Source: three-view drawing plus pictorial views. Frame: mm from the lowest corner of the part. Give positions to 0.01 mm unless a question says otherwise; leave off trailing zeros. Write each loop counter-clockwise with the first axis right and the second up, starting at its lowest first coordinate (ties: lowest second). Pieces come first, ordered by that corner, then holes. Notation, with made-up numbers: (12, 18) -> (23, 18) arc R29 cw to (23, 55) -> close; hole circle Ø8 at (5, 42.25). An arc over 180 degrees is marked (long way). Write item = value, one per line.
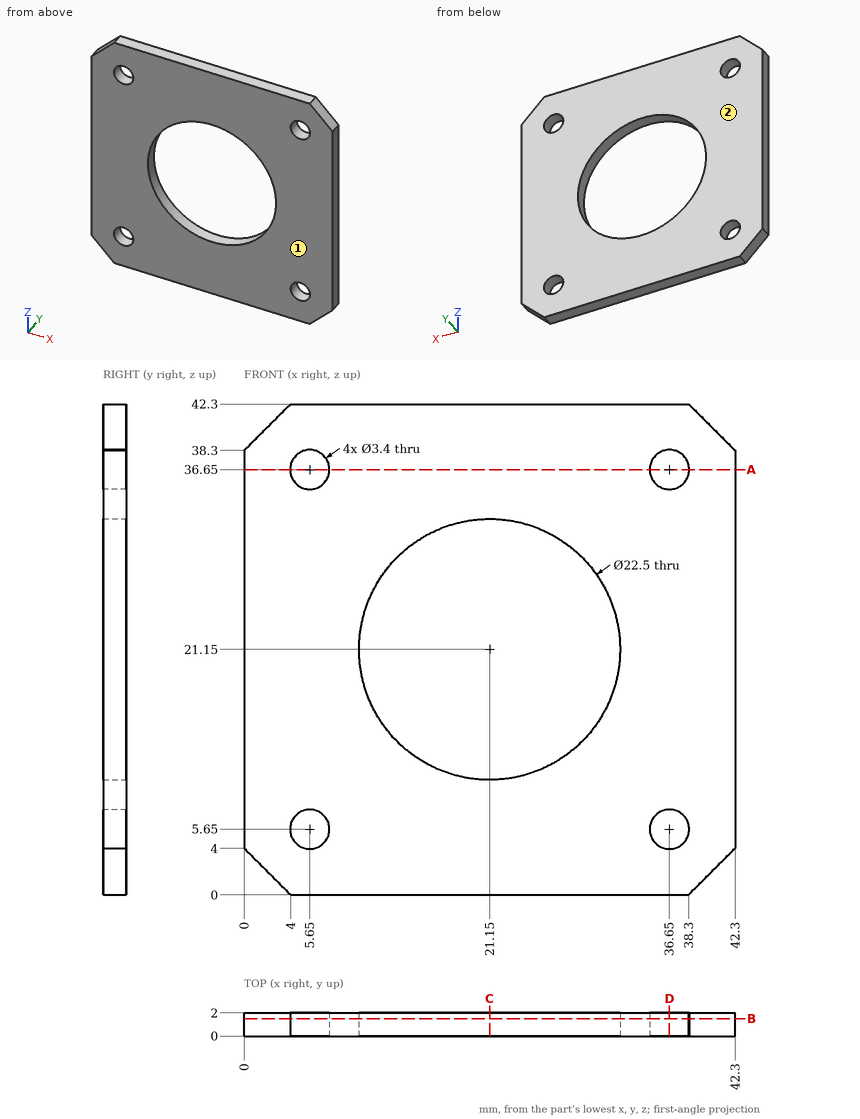
1) Cut plane D-D (x = 36.65). Return the cut outline in (y, z), then the cut area to 3 significant figures.
Computed:
outline = (0, 0) -> (2, 0) -> (2, 3.95) -> (0, 3.95) -> close; (0, 7.35) -> (2, 7.35) -> (2, 34.95) -> (0, 34.95) -> close; (0, 38.35) -> (2, 38.35) -> (2, 42.3) -> (0, 42.3) -> close
area = 71.0 mm²
2) Contact query for a flat-ended pin moving along its axis: pin 1 (2 mm diameter, centred on x = 5.65, z = 36.65, fed in from -Y). Output: stop coordinate, or through.
Computed:
pin_1 = through
3) Cut plane A-A (z = 36.65). Return the cut outline in (x, y), then the cut area to 3 significant figures.
Computed:
outline = (0, 0) -> (3.95, 0) -> (3.95, 2) -> (0, 2) -> close; (7.35, 0) -> (34.95, 0) -> (34.95, 2) -> (7.35, 2) -> close; (38.35, 0) -> (42.3, 0) -> (42.3, 2) -> (38.35, 2) -> close
area = 71.0 mm²
4) Material intervals for L1, parallel to Z at x = 5.65, y = 1.3; L2, parallel to X at y = 0.2, z = 21.5, sorted ascending.
Computed:
L1 = 0 to 3.95, 7.35 to 34.95, 38.35 to 42.3
L2 = 0 to 9.91, 32.39 to 42.3
5) Cut plane B-B (y = 1.5). Return the cut outline in (x, z), then the cut area to 3 significant figures.
Computed:
outline = (0, 4) -> (4, 0) -> (38.3, 0) -> (42.3, 4) -> (42.3, 38.3) -> (38.3, 42.3) -> (4, 42.3) -> (0, 38.3) -> close; hole circle Ø3.4 at (5.65, 5.65); hole circle Ø3.4 at (5.65, 36.65); hole circle Ø22.5 at (21.15, 21.15); hole circle Ø3.4 at (36.65, 5.65); hole circle Ø3.4 at (36.65, 36.65)
area = 1,320 mm²
6) Draft query along Y for the marked faces 1 and 2. Return one class per face: pulls with the +Y half, pulls with the -Y half, needs draft (parallel to the pull), parting line crosses it, or undercut.
Computed:
face_1 = pulls with the -Y half
face_2 = pulls with the +Y half
7) Cut plane C-C (x = 21.15). Return the cut outline in (y, z).
Computed:
outline = (0, 0) -> (2, 0) -> (2, 9.9) -> (0, 9.9) -> close; (0, 32.4) -> (2, 32.4) -> (2, 42.3) -> (0, 42.3) -> close
